```python
from build123d import *

# Parameters (mm, degrees)
SKETCH_W        = 213
SKETCH_H        = 360
PAD_DEPTH       = 6.5
SKETCH001_R     = 5.2
POCKET_DEPTH    = 3.4
SKETCH002_R     = 3.2
POCKET001_DEPTH = 3.1
FILLET_R        = 4
SKETCH003_W     = 160
SKETCH003_H     = 80
POCKET002_DEPTH = 6.5
FILLET001_R     = 4
FILLET002_R     = 4


with BuildPart() as part:
    # Sketch → Pad (new body)
    with BuildSketch(Plane.XY):
        with Locations((106.5, 180)):
            Rectangle(SKETCH_W, SKETCH_H)
    extrude(amount=PAD_DEPTH)

    # Sketch001 (on Face6 of Pad) → Pocket (cut)
    with BuildSketch(Plane.XY.offset(6.5)):
        with Locations((106.5, 350)):
            Circle(SKETCH001_R)
        with Locations((16.5, 240)):
            Circle(SKETCH001_R)
        with Locations((16.5, 120)):
            Circle(SKETCH001_R)
        with Locations((196.5, 240)):
            Circle(SKETCH001_R)
        with Locations((196.5, 120)):
            Circle(SKETCH001_R)
        with Locations((106.5, 10)):
            Circle(SKETCH001_R)
    extrude(amount=-POCKET_DEPTH, mode=Mode.SUBTRACT)

    # Sketch002 (on Face17 of Pocket) → Pocket001 (cut)
    with BuildSketch(Plane.XY.offset(3.1)):
        with Locations((106.5, 350)):
            Circle(SKETCH002_R)
        with Locations((16.5, 240)):
            Circle(SKETCH002_R)
        with Locations((16.5, 120)):
            Circle(SKETCH002_R)
        with Locations((196.5, 240)):
            Circle(SKETCH002_R)
        with Locations((196.5, 120)):
            Circle(SKETCH002_R)
        with Locations((106.5, 10)):
            Circle(SKETCH002_R)
    extrude(amount=-POCKET001_DEPTH, mode=Mode.SUBTRACT)

    # Fillet
    fillet_edges = [part.edges().sort_by_distance(p)[0] for p in [
        (213, 180, 6.5),
        (0, 180, 6.5),
    ]]
    fillet(fillet_edges, radius=FILLET_R)

    # Sketch003 (on Face5 of Fillet) → Pocket002 (cut)
    with BuildSketch(Plane.XY.offset(6.5)):
        with Locations((106.5, 260)):
            Rectangle(SKETCH003_W, SKETCH003_H)
    extrude(amount=-POCKET002_DEPTH, mode=Mode.SUBTRACT)

    # Fillet001
    fillet001_edges = [part.edges().sort_by_distance(p)[0] for p in [
        (26.5, 220, 3.25),
    ]]
    fillet(fillet001_edges, radius=FILLET001_R)

    # Fillet002
    fillet002_edges = [part.edges().sort_by_distance(p)[0] for p in [
        (186.5, 220, 3.25),
        (186.5, 300, 3.25),
        (26.5, 300, 3.25),
    ]]
    fillet(fillet002_edges, radius=FILLET002_R)


solid = part.part
```
Verification items for the finished model (mm, model axes). A direction names the side the tool comes from. Coordinates: 2 decimals unless noted, no trailing zeros. Loops run counter-clockwise (first coordinate to the right, second up) from the corner with the lowest first, then second, coordinate; pieces in that order, holes last. Notation, with made-up numbers: (65.25, -15.75) -> (109.25, -15.75) arc R14 ccw to (109.25, -8.75) -> close; hole circle Ø11 at (28.25, 71.5). An arc over 180 degrees is marked (long way). Answer in a Markdown table with one row per item. Add a question column.
1. Section check C-C, the plane z = 1.5. Enter the section's corners in (x, y), then the cut area to 3 significant figures.
2. Draft check along Y on faces 1 (the face through (105, 183, 0)), 2 (the face through (105, 0, 3)), 3 (the face through (105, 360, 3)), 4 (the face through (19.3, 244.38, 4.82)). Enter one of: +Y half, -Y half, draft (parallel to the pull), parting line (faces both ways), or undercut.
3. Access from +Z, -Z, +X, -X, +Y, -Y to the whole of each face (thin tool, end or side, straight path). Record for faces 5 (the face through (101.305, 10.229, 4.824)), 6 (the face through (26.5, 259, 3)).
4. Section check B-B, the plane x = 37. Enter the section's corners in (y, z).
5. Depth check by flat-ended pin: P1, Ø2, axis at x = 69, z = 3, coming from the -Y side; P2, Ø1, axis at y = 280.5, z = 5, coming from the -X side; P3, Ø9.5, axis at x = 16.5, y = 120, coming from the +Z side. Enter the tip coordinate at first touch or a pass-through.
6. Material ranges on probe 1 along Y at (x, z) = (16.5, 1); probe 2 along Y at (x, z) = (106.5, 1.55); probe 3 along Y at (x, z) = (144, 0.5), recorded low to high. Write a range as [from, to].
7. Section check A-A, the plane y = 287.5. Enter the section's corners in (x, z).
Derived:
| question | item | result |
|---|---|---|
| 1 | outline | (0, 0) -> (213, 0) -> (213, 360) -> (0, 360) -> close; hole circle Ø6.4 at (16.5, 120); hole circle Ø6.4 at (16.5, 240); hole (26.5, 224) arc R4 ccw to (30.5, 220) -> (182.5, 220) arc R4 ccw to (186.5, 224) -> (186.5, 296) arc R4 ccw to (182.5, 300) -> (30.5, 300) arc R4 ccw to (26.5, 296) -> close; hole circle Ø6.4 at (106.5, 10); hole circle Ø6.4 at (106.5, 350); hole circle Ø6.4 at (196.5, 120); hole circle Ø6.4 at (196.5, 240) |
| 1 | area | 63,700 mm² |
| 2 | face 1 | draft |
| 2 | face 2 | -Y half |
| 2 | face 3 | +Y half |
| 2 | face 4 | undercut |
| 3 | face 5 | +Z |
| 3 | face 6 | +Z, -Z |
| 4 | outline | (0, 0) -> (220, 0) -> (220, 6.5) -> (0, 6.5) -> close; (300, 0) -> (360, 0) -> (360, 6.5) -> (300, 6.5) -> close |
| 5 | P1 | stops at y = 0 |
| 5 | P2 | stops at x = 0.54 |
| 5 | P3 | stops at z = 3.1 |
| 6 | probe 1 | y = [0, 116.8], [123.2, 236.8], [243.2, 360] |
| 6 | probe 2 | y = [0, 6.8], [13.2, 220], [300, 346.8], [353.2, 360] |
| 6 | probe 3 | y = [0, 220], [300, 360] |
| 7 | outline | (0, 0) -> (26.5, 0) -> (26.5, 6.5) -> (4, 6.5) arc R4 ccw to (0, 2.5) -> close; (186.5, 0) -> (213, 0) -> (213, 2.5) arc R4 ccw to (209, 6.5) -> (186.5, 6.5) -> close |
